```python
from build123d import *

# Parameters (mm, degrees)
F0_R            = 50.8
F1_DEPTH        = 25.4
F2_R            = 6.35
F3_DEPTH        = 25.4
F3_COPIES_COUNT = 12
F5_DEPTH        = 25.4
F5_COPIES_COUNT = 24


# Not quite as in the source:
# - a pattern or mirror of a feature is missing from the dataset's text; its kind, count and spacing are read off the source's solid


with BuildPart() as f1:
    # F0 (on Top) → F1 (new body)
    with BuildSketch(Plane.XY):
        Circle(F0_R)
    extrude(amount=F1_DEPTH)

    # F2 (on face) → F3 (join)
    with BuildSketch(Plane.XY.offset(25.4)):
        with Locations((-27.5896564126, 26.2101721019)):
            Circle(F2_R)
    f3 = extrude(amount=F3_DEPTH)

    # F3_copies: F3 ×12 about axis
    f3_copies_axis = Axis((0, 0, 0), (0, 0, 1))
    for i in range(1, F3_COPIES_COUNT):
        add(f3.rotate(f3_copies_axis, i * 360 / F3_COPIES_COUNT))

    # F4 (on face) → F5 (join)
    with BuildSketch(Plane.XY.offset(25.4)):
        with BuildLine():
            Line((4.8960702354, 50.5635095326), (0, 58.7265528738))
            Line((0, 58.7265528738), (-4.8960702354, 50.5635095326))
            ThreePointArc((-4.8960702354, 50.5635095326), (0, 50.8), (4.8960702354, 50.5635095326))
        make_face()
        with BuildLine():
            Line((4.8960702354, 50.5635095326), (-4.8960702354, 50.5635095326))
            ThreePointArc((-4.8960702354, 50.5635095326), (-34.1461537515, -37.6122344986), (50.8, 0))
            ThreePointArc((50.8, 0), (37.6122344986, 34.1461537515), (4.8960702354, 50.5635095326))
        make_face()
        with BuildLine():
            ThreePointArc((4.8960702354, 50.5635095326), (0, 50.8), (-4.8960702354, 50.5635095326))
            Line((-4.8960702354, 50.5635095326), (4.8960702354, 50.5635095326))
        make_face()
    f5 = extrude(amount=-F5_DEPTH)

    # F5_copies: F5 ×24 about axis
    f5_copies_axis = Axis((0, 0, 0), (0, 0, 1))
    for i in range(1, F5_COPIES_COUNT):
        add(f5.rotate(f5_copies_axis, i * 360 / F5_COPIES_COUNT))


solid = f1.part
```
Can you work these out from the model? Positions are in its coordinate system, mm. A direction names the side the tool comes from. Coordinates: 2 decimals unless noted, no trailing zeros. Order: outer loops, then holes, each group sorted by start corner. A loop starts at its lowest first (then second) coordinate and runs counter-clockwise, first axis right, second up. Notation, with made-up numbers: (-17.75, 42) -> (-8.75, 42) arc R14 ccw to (-8.75, 66) -> close; hole circle Ø9 at (20, 12). An arc over 180 degrees is marked (long way). Write each question's results on one line, items separated by ' | '.
Item 1: I want a section at A-A, the plane z = 41. Count the separate pieces of the cut face and the enclosed holes in it, then the cut area to 3 significant figures.
Results are:
separate pieces: 12 | enclosed holes: 0 | area: 1,520 mm²
Item 2: If we mould it in two halves opening along X, with no side actions, what happens to faces 1 (the face through (-48.516, -25.144, 12.878)), 2 (the face through (-28, 26, 50.8)), 3 (the face through (-11.73, 53.37, 12.88))? For each: +X half, -X half, draft (parallel to the pull), parting line (faces both ways), or undercut.
Results are:
face 1: -X half | face 2: draft | face 3: undercut
Item 3: Which directions (+Z, -Z, +X, -X, +Y, -Y) give clear straight access to the entire face, cutting with the end or side of a thin tool? Please do faces 4 (the face through (-16.49, 52.21, 12.88)), 5 (the face through (-19.463, -46.924, 12.878)), 6 (the face through (-3.04, -39.43, 37.92)), 7 (the face through (-54.59, 2.48, 12.88)), 8 (the face through (53.37, 11.73, 12.88)).
Results are:
face 4: +Z, -Z, +Y | face 5: +Z, -Z, -Y | face 6: +Z | face 7: +Z, -Z, -X | face 8: +Z, -Z, +X
Item 4: I'm going to push flat-ended pins straight in: pin 1 Ø4 at (y, z) = (-22.5, 34.5) entering from -X; pin 2 Ø2 at (y, z) = (8, 13.5) entering from +X; pin 3 Ø3 at (x, z) = (0.5, 32) entering from +Y; pin 4 Ø3 at (x, y) = (-40.5, 35) entering from +Z. Where does each tip first touch, or does it pass through?
Results are:
pin 1: x = -31.76 | pin 2: x = 50.73 | pin 3: through | pin 4: z = 25.4
Item 5: I want a section at B-B, the plane y = 10.5. Write out the boundary of the cut face in (x, z).
Results are:
outline: (-52.18, 0) -> (52.18, 0) -> (52.18, 25.4) -> (42.84, 25.4) -> (42.84, 50.8) -> (30.15, 50.8) -> (30.15, 25.4) -> (-30.85, 25.4) -> (-30.85, 50.8) -> (-43.14, 50.8) -> (-43.14, 25.4) -> (-52.18, 25.4) -> close
Item 6: I want a section at C-C, the plane x = -36.5. Write out the boundary of the cut face in (y, z), then the cut area to 3 significant figures.
Results are:
outline: (-40.27, 0) -> (40.27, 0) -> (40.27, 25.4) -> (15.23, 25.4) -> (15.23, 50.8) -> (2.57, 50.8) -> (2.57, 25.4) -> (-4.44, 25.4) -> (-4.44, 50.8) -> (-17.14, 50.8) -> (-17.14, 25.4) -> (-40.27, 25.4) -> close | area: 2,690 mm²
Item 7: If I drill on line 1 along Y through (x, z) = (51, 15.5); line 2 along X through (y, z) = (37, 40); line 3 along Z through (x, y) = (-18, -22), over which ranges is the centre line in solid material (lowest first)?
Results are:
line 1: -16.84 to -9.28, -4.63 to 4.63, 9.28 to 16.84 | line 2: -17.12 to -4.46, 2.55 to 15.25 | line 3: 0 to 25.4
